Part model, mm, in its own coordinate system. A direction names the side the tool comes from. Give positions to 0.01 mm unless a question says otherwise; leave off trailing zeros. Order: outer loops, then holes, each group sorted by start corner. A loop starts at its lowest first (then second) coordinate and runs counter-clockwise, first axis right, second up.
1. Slice it at C-C on x = 0.4. List the corners of the cut face in (y, z).
2. Drop a flat-ended pin along its axis: pin 1 Ø2 at (x, y) = (-0.5, 3.5) entering from +Z. Give the stop position or say it passes through.
3. Mould opens along X. For faces 3 (the flat face through (2.5, 2, 2)), 4 (the flat face through (-2, 4.762, 2)), 5 (the flat face through (1, 3, 2)) say: +X half, -X half, draft (parallel to the pull), parting line (faces both ways), or undercut.
4. Which spindle directions (+Z, -Z, +X, -X, +Y, -Y) get a long thin tool onto all of the face, cutting with end or side? Do faces 1 (the flat face through (0, -0.762, 2)), 2 (the flat face through (0, 1.962, 2)). Say none if no direction does.
5. Probe line 1 (X direction, y = 2.6, z = 2.75); line 2 (Y direction, x = 0.8, z = 1.3). List the from-to ranges inside material, lowest first.
6. Slice it at A-A on y = 4.2. List the corners of the cut face in (x, z), and give its area (3 significant figures).
7. Slice it at B-B on z = 1.95. List the corners of the cut face in (x, y).
from build123d import *

# Parameters (mm, degrees)
SKETCH1_W           = 5
SKETCH1_H           = 1.524
BOSS_EXTRUDE1_DEPTH = 4.0259


with BuildPart() as part:
    # Sketch1 → Boss-Extrude1 (new body)
    with BuildSketch(Plane.XY):
        Polygon((-1, 1.962), (-1, 4.762), (-2.5, 4.762), (-2.5, 0.762), (2.5, 0.762), (2.5, 4.762), (1, 4.762), (1, 1.962), align=None)
        Rectangle(SKETCH1_W, SKETCH1_H)
    extrude(amount=BOSS_EXTRUDE1_DEPTH)


solid = part.part
Data:
1. outline: (-0.76, 0) - (1.96, 0) - (1.96, 4.03) - (-0.76, 4.03) - close
2. pin 1: stops at z = 4.03
3. face 3: +X half
3. face 4: draft
3. face 5: undercut
4. face 1: +Z, -Z, +X, -X, -Y
4. face 2: +Z, -Z, +Y
5. line 1: x = -2.5 to -1, 1 to 2.5
5. line 2: y = -0.76 to 1.96
6. outline: (-2.5, 0) - (-1, 0) - (-1, 4.03) - (-2.5, 4.03) - close; (1, 0) - (2.5, 0) - (2.5, 4.03) - (1, 4.03) - close
6. area: 12.1 mm2
7. outline: (-2.5, -0.76) - (2.5, -0.76) - (2.5, 4.76) - (1, 4.76) - (1, 1.96) - (-1, 1.96) - (-1, 4.76) - (-2.5, 4.76) - close
